The model under review builds one solid part; all positions refer to its coordinate system, in mm. Face numbers are marked on the shaded views. A direction names the side the tool comes from. Coordinates: 2 decimals unless noted, no trailing zeros. Write each loop counter-clockwise with the first axis right and the second up, starting at its lowest first coordinate (ties: lowest second). Pieces come first, ordered by that corner, then holes.
1) For P1, Ø6, axis at x = 16, y = -10, coming from the -Z side, flat-tipped, find the tip position at first contact; note if it passes through.
2) Machinability: for the marked faces 1 and 2, which of the approach directions +Z, -Z, +X, -X, +Y, -Y give a long, thin tool a straight path to every point of the face, cutting with its end or side? Answer none if there is none.
3) Add section A-A, the plane x = 7. State the section outline as (y, z) points (3 decimals).
4) For line 1 (Y direction, x = 5, z = 27.5); line 2 (Z direction, x = 17.25, y = -32) (3 decimals); line 3 (X direction, y = -24, z = 12.5), list the stretches that pass through material, from the lowest coordinate up.
from build123d import *

# Parameters (mm, degrees)
F1_DEPTH     = 25
F2_T1_DEPTH  = 50.5172412843
F2_T3_DEPTH  = 43.0387943983
F2_T5_DEPTH  = 33.0603428185
F2_T7_DEPTH  = 41.8750006706
F2_T13_DEPTH = 63.0172412843
F2_T17_DEPTH = 45.5603428185


# Not quite as in the source:
# - a fillet or chamfer that OpenCascade refuses, or shapes differently, is made with other operations: its cross-section is extruded or revolved along the edge and cut away or added


with BuildPart() as f1:
    # F0 (on Right) → F1 (new body)
    with BuildSketch(Plane.YZ):
        Polygon((-38.5991372168, 16.8750006706), (-38.5991372168, 0), (0, 0), (0, 54.8922419548), (-18.0387943983, 54.8922419548), (-18.0387943983, 16.8750006706), align=None)
    extrude(amount=F1_DEPTH)

    # F2: fillet of radius 5 on 4 edges, made by hand

    # F2_s2 → F2_t1 (cut)
    with BuildSketch(Plane.XY.offset(16.8750006706)):
        with BuildLine():
            add(Edge.make_bspline(
                [(20, -18.0387943983), (25, -18.0387943983), (25, -13.0387943983)],
                knots=[0, 0, 0, 1, 1, 1], degree=2, weights=[1, 1, 1]))
            Line((25, -13.0387943983), (25, -18.0387943983))
            Line((25, -18.0387943983), (20, -18.0387943983))
        make_face()
    extrude(amount=F2_T1_DEPTH, mode=Mode.SUBTRACT)

    # F2_s4 → F2_t3 (cut)
    with BuildSketch(Plane.XZ.offset(-12.5)):
        with BuildLine():
            add(Edge.make_bspline(
                [(20, 54.8922419548), (25, 54.8922419548), (25, 49.8922419548)],
                knots=[0, 0, 0, 1, 1, 1], degree=2, weights=[1, 1, 1]))
            Line((25, 49.8922419548), (25, 54.8922419548))
            Line((25, 54.8922419548), (20, 54.8922419548))
        make_face()
    extrude(amount=F2_T3_DEPTH, mode=Mode.SUBTRACT)

    # F2_s6 → F2_t5 (cut)
    with BuildSketch(Plane.XZ.offset(18.0387943983)):
        with BuildLine():
            add(Edge.make_bspline(
                [(20, 16.8750006706), (25, 16.8750006706), (25, 11.8750006706)],
                knots=[0, 0, 0, 1, 1, 1], degree=2, weights=[1, 1, 1]))
            Line((25, 11.8750006706), (25, 16.8750006706))
            Line((25, 16.8750006706), (20, 16.8750006706))
        make_face()
    extrude(amount=F2_T5_DEPTH, mode=Mode.SUBTRACT)

    # F2_s8 → F2_t7 (cut)
    with BuildSketch(Plane.XY.offset(-12.5)):
        with BuildLine():
            add(Edge.make_bspline(
                [(20, -38.5991372168), (25, -38.5991372168), (25, -33.5991372168)],
                knots=[0, 0, 0, 1, 1, 1], degree=2, weights=[1, 1, 1]))
            Line((25, -33.5991372168), (25, -38.5991372168))
            Line((25, -38.5991372168), (20, -38.5991372168))
        make_face()
    extrude(amount=F2_T7_DEPTH, mode=Mode.SUBTRACT)


with BuildPart() as f2_tool11:
    # F2_s12 → F2_t13 (new body)
    with BuildSketch(Plane.XY.offset(67.3922419548)):
        with BuildLine():
            add(Edge.make_bspline(
                [(20, -18.0387943983), (25, -18.0387943983), (25, -13.0387943983)],
                knots=[0, 0, 0, 1, 1, 1], degree=2, weights=[1, 1, 1]))
            Line((25, -13.0387943983), (25, -18.0387943983))
            Line((25, -18.0387943983), (20, -18.0387943983))
        make_face()
    extrude(amount=-F2_T13_DEPTH)

    split(bisect_by=Plane.XY.offset(16.8750006706), keep=Keep.BOTTOM)


with BuildPart() as f2_tool15:
    # F2_s16 → F2_t17 (new body)
    with BuildSketch(Plane.XZ.offset(5.5387943983)):
        with BuildLine():
            add(Edge.make_bspline(
                [(20, 16.8750006706), (25, 16.8750006706), (25, 11.8750006706)],
                knots=[0, 0, 0, 1, 1, 1], degree=2, weights=[1, 1, 1]))
            Line((25, 11.8750006706), (25, 16.8750006706))
            Line((25, 16.8750006706), (20, 16.8750006706))
        make_face()
    extrude(amount=F2_T17_DEPTH)

    split(bisect_by=Plane.XZ.offset(18.0387943983), keep=Keep.BOTTOM)


with BuildPart() as f2_tool11_1:
    add(f2_tool11.part)

    # F2_t19: intersect F2_tool15
    add(f2_tool15.part, mode=Mode.INTERSECT)


with BuildPart() as f1_1:
    add(f1.part)

    # F2_t9: cut F2_tool11
    add(f2_tool11_1.part, mode=Mode.SUBTRACT)


solid = f1_1.part
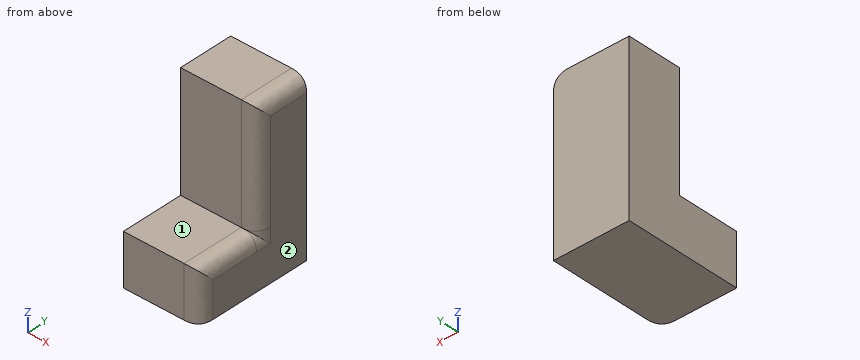
Geometry results:
1. P1: stops at z = 0
2. face 1: +Z, +X, -X, -Y
2. face 2: +Z, -Z, +X, +Y, -Y
3. outline: (-38.599, 0) - (0, 0) - (0, 54.892) - (-18.039, 54.892) - (-18.039, 16.875) - (-38.599, 16.875) - close
4. line 1: y = -18.04 to 0
4. line 2: z = 0 to 16.875
4. line 3: x = 0 to 24.98
